Here's how the part is built. I have some questions about the finished solid (model axes, mm). A direction names the side the tool comes from. Coordinates: 2 decimals unless noted, no trailing zeros. Order: outer loops, then holes, each group sorted by start corner. A loop starts at its lowest first (then second) coordinate and runs counter-clockwise, first axis right, second up. Notation, with made-up numbers: (14.5, 13.5) - (70.5, 13.5) arc R22 ccw to (70.5, 26.5) - close; hole circle Ø10 at (26.5, -7). An arc over 180 degrees is marked (long way). Answer as CSV lines item,"result". Start each with the question number.
Q1. Suppose I cut it at B-B (x = 6). Please give me the cut outline in (y, z), then the cut area to 3 significant figures.
Q2. For faces 5 (the face through (4.5, 25, 8)), 6 (the face through (9.5, 24, 11)), 7 (the face through (13, 0, 0)), which set-ups out of +Z, -Z, +X, -X, +Y, -Y let a thin tool reach every point of the face, with its end or its side?
Q3. Suppose I cut it at A-A (x = -15). Please give me the cut outline in (y, z).
Q4. Thinking about a two-plate mould opening in Y: for faces 1 (the face through (-0.3, 8.3, -5)), 2 (the face through (0.08, 18.3, 10.51)), 3 (the face through (16.669, -30.526, -2.535)), 4 (the face through (-7, 30, 18)), which applies, released by +Y, released by -Y, zero draft, split by the parting line, or undercut?
Q5. For pin 1 Ø8.5 at (y, z) = (17.5, 20) entering from +X; pin 2 Ø11 at (y, z) = (-9.5, 18) entering from +X; pin 3 Ø5.5 at (x, z) = (-6.5, 23) entering from +Y; pin 4 Ø3 at (x, y) = (-15, 30) entering from -Z, each with a flat end and sliding along its axis, tell me the tip position at first contact or that it passes through.
Q6. I need wall thicknesses on line 1 (Y direction, x = 15, z = -2); line 2 (Z direction, x = -13, y = -27); line 3 (X direction, y = 19.5, z = 20.5). Which ranges of each line are inside material? Lowest first, please.
from build123d import *

# Parameters (mm, degrees)
SKETCH_1_W                           = 40
SKETCH_1_H                           = 70
EXTRUDE_1_DEPTH                      = 5
EXTRUDE_2_REACH                      = 92.62
EXTRUDE_START                        = -50
SKETCH_2_R                           = 12
CUT_EXTRUDE_1_REACH                  = 69.832
SKETCH_4_R                           = 1.75
FILLET_1_R                           = 3
EXTRUDE_START_2                      = 7
EXTRUDE_3_DEPTH                      = 2.5
EXTRUDE_START_3                      = -7
EXTRUDE_4_DEPTH                      = 2.5
SKETCH_5_R                           = 9.4
CUT_EXTRUDE_2_DEPTH                  = 80.580228084
CUT_EXTRUDE_3_REACH                  = 65.9
CUT_EXTRUDE_3_END_RADIUS             = 12
SKETCH_7_R                           = 1.75
CUT_EXTRUDE_3_DIRECTION_2_REACH      = 65.9
CUT_EXTRUDE_3_DIRECTION_2_END_RADIUS = 12


with BuildPart() as part:
    # ｽｹｯﾁ1 → ﾎﾞｽ - 押し出し1 (new body)
    with BuildSketch(Plane.XY):
        Rectangle(SKETCH_1_W, SKETCH_1_H)
    extrude(amount=-EXTRUDE_1_DEPTH)

    # ﾎﾞｽ - 押し出し2: up to this plane
    extrude_2_end = Plane(origin=(0, 0, 0), z_dir=(0, 0, 1))
    # ｽｹｯﾁ2 → ﾎﾞｽ - 押し出し2 (add, up to the surface)
    with BuildSketch(Plane(origin=(0, 0, 0), x_dir=(1, 0, 0), z_dir=(0, -0.49999999999999495, -0.8660254037844416)).offset(EXTRUDE_START), mode=Mode.PRIVATE) as extrude_2_sk1:
        with Locations(Location((0, 0, 0), (0, 0, 270))):
            Circle(SKETCH_2_R)
    extrude_2_tool1 = split(extrude(extrude_2_sk1.sketch, amount=EXTRUDE_2_REACH, mode=Mode.PRIVATE), bisect_by=extrude_2_end, keep=Keep.BOTH, mode=Mode.PRIVATE)
    add(extrude_2_tool1.solids().sort_by_distance((0, 25, 43.30127))[0])

    # ｽｹｯﾁ4 → ｶｯﾄ - 押し出し1 (cut, up to next)
    with BuildSketch(Plane(origin=(0, 0, -5), x_dir=(-1, 0, 0), z_dir=(0, 0, -1)), mode=Mode.PRIVATE) as cut_extrude_1_sk1:
        with Locations((-15, 30)):
            Circle(SKETCH_4_R)
    cut_extrude_1_tool1 = extrude(cut_extrude_1_sk1.sketch, amount=-CUT_EXTRUDE_1_REACH, mode=Mode.PRIVATE) & part.part
    # ｽｹｯﾁ4 → ｶｯﾄ - 押し出し1 (cut, up to next)
    with BuildSketch(Plane(origin=(0, 0, -5), x_dir=(-1, 0, 0), z_dir=(0, 0, -1)), mode=Mode.PRIVATE) as cut_extrude_1_sk2:
        with Locations(Location((15, 30, 0), (0, 0, 180))):
            Circle(SKETCH_4_R)
    cut_extrude_1_tool2 = extrude(cut_extrude_1_sk2.sketch, amount=-CUT_EXTRUDE_1_REACH, mode=Mode.PRIVATE) & part.part
    # ｽｹｯﾁ4 → ｶｯﾄ - 押し出し1 (cut, up to next)
    with BuildSketch(Plane(origin=(0, 0, -5), x_dir=(-1, 0, 0), z_dir=(0, 0, -1)), mode=Mode.PRIVATE) as cut_extrude_1_sk3:
        with Locations((15, -30)):
            Circle(SKETCH_4_R)
    cut_extrude_1_tool3 = extrude(cut_extrude_1_sk3.sketch, amount=-CUT_EXTRUDE_1_REACH, mode=Mode.PRIVATE) & part.part
    # ｽｹｯﾁ4 → ｶｯﾄ - 押し出し1 (cut, up to next)
    with BuildSketch(Plane(origin=(0, 0, -5), x_dir=(-1, 0, 0), z_dir=(0, 0, -1)), mode=Mode.PRIVATE) as cut_extrude_1_sk4:
        with Locations(Location((-15, -30, 0), (0, 0, 180))):
            Circle(SKETCH_4_R)
    cut_extrude_1_tool4 = extrude(cut_extrude_1_sk4.sketch, amount=-CUT_EXTRUDE_1_REACH, mode=Mode.PRIVATE) & part.part
    add(cut_extrude_1_tool1.solids().sort_by_distance((15, 30, -5))[0], mode=Mode.SUBTRACT)
    add(cut_extrude_1_tool2.solids().sort_by_distance((-15, 30, -5))[0], mode=Mode.SUBTRACT)
    add(cut_extrude_1_tool3.solids().sort_by_distance((-15, -30, -5))[0], mode=Mode.SUBTRACT)
    add(cut_extrude_1_tool4.solids().sort_by_distance((15, -30, -5))[0], mode=Mode.SUBTRACT)

    # ﾌｨﾚｯﾄ1
    fillet_1_edges = [part.edges().sort_by_distance(p)[0] for p in [
        (20, -35, -2.5),
        (-20, -35, -2.5),
        (-20, 35, -2.5),
        (20, 35, -2.5),
    ]]
    fillet(fillet_1_edges, radius=FILLET_1_R)

    # ｽｹｯﾁ6 → ﾎﾞｽ - 押し出し3 (add, symmetric)
    with BuildSketch(Plane(origin=(0, 0, 0), x_dir=(0, 0, -1), z_dir=(1, 0, 0)).offset(EXTRUDE_START_2)):
        Polygon((0, 30), (-38, 30), (-38, 14), (0, -30), align=None)
    extrude(amount=EXTRUDE_3_DEPTH, both=True)

    # ｽｹｯﾁ6<2> → ﾎﾞｽ - 押し出し4 (add, symmetric)
    with BuildSketch(Plane(origin=(0, 0, 0), x_dir=(0, 0, -1), z_dir=(1, 0, 0)).offset(EXTRUDE_START_3)):
        Polygon((0, 30), (-38, 30), (-38, 14), (0, -30), align=None)
    extrude(amount=EXTRUDE_4_DEPTH, both=True)

    # ｽｹｯﾁ5 → ｶｯﾄ - 押し出し2 (cut, through all)
    with BuildSketch(Plane(origin=(0, 25, 43.301270189), x_dir=(1, 0, 0), z_dir=(0, 0.49999999999999495, 0.8660254037844416))):
        with Locations(Location((0, 0, 0), (0, 0, 270))):
            Circle(SKETCH_5_R)
    extrude(amount=-CUT_EXTRUDE_2_DEPTH, mode=Mode.SUBTRACT)

    # ｶｯﾄ - 押し出し3: up to this cylinder (the profile starts inside it)
    cut_extrude_3_end = Plane(origin=(0, 14.999999951, 25.980762028), z_dir=(0, 0.4999999999999949, 0.8660254037844416)) * Cylinder(CUT_EXTRUDE_3_END_RADIUS, 176.799999934, mode=Mode.PRIVATE)
    # ｽｹｯﾁ7 → ｶｯﾄ - 押し出し3 (cut, up to the surface)
    with BuildSketch(Plane(origin=(0, 0, 0), x_dir=(1, 0, 0), z_dir=(0, 0.8660254037844416, -0.49999999999999495)), mode=Mode.PRIVATE) as cut_extrude_3_sk1:
        with Locations(Location((0, -20, 0), (0, 0, 270))):
            Circle(SKETCH_7_R)
    cut_extrude_3_tool1 = extrude(cut_extrude_3_sk1.sketch, amount=-CUT_EXTRUDE_3_REACH, mode=Mode.PRIVATE) & cut_extrude_3_end
    add(cut_extrude_3_tool1.solids().sort_by_distance((0, 10, 17.320508))[0], mode=Mode.SUBTRACT)
    # ｽｹｯﾁ7 → ｶｯﾄ - 押し出し3 (cut, up to the surface)
    with BuildSketch(Plane(origin=(0, 0, 0), x_dir=(1, 0, 0), z_dir=(0, 0.8660254037844416, -0.49999999999999495)), mode=Mode.PRIVATE) as cut_extrude_3_sk2:
        with Locations(Location((0, -40, 0), (0, 0, 270))):
            Circle(SKETCH_7_R)
    cut_extrude_3_tool2 = extrude(cut_extrude_3_sk2.sketch, amount=-CUT_EXTRUDE_3_REACH, mode=Mode.PRIVATE) & cut_extrude_3_end
    add(cut_extrude_3_tool2.solids().sort_by_distance((0, 20, 34.641016))[0], mode=Mode.SUBTRACT)

    # ｶｯﾄ - 押し出し3 direction 2: up to this cylinder (the profile starts inside it)
    cut_extrude_3_direction_2_end = Plane(origin=(0, 14.999999951, 25.980762028), z_dir=(0, 0.4999999999999949, 0.8660254037844416)) * Cylinder(CUT_EXTRUDE_3_DIRECTION_2_END_RADIUS, 176.799999934, mode=Mode.PRIVATE)
    # ｽｹｯﾁ7 → ｶｯﾄ - 押し出し3 direction 2 (cut, up to the surface)
    with BuildSketch(Plane(origin=(0, 0, 0), x_dir=(1, 0, 0), z_dir=(0, 0.8660254037844416, -0.49999999999999495)), mode=Mode.PRIVATE) as cut_extrude_3_direction_2_sk1:
        with Locations(Location((0, -20, 0), (0, 0, 270))):
            Circle(SKETCH_7_R)
    cut_extrude_3_direction_2_tool1 = extrude(cut_extrude_3_direction_2_sk1.sketch, amount=CUT_EXTRUDE_3_DIRECTION_2_REACH, mode=Mode.PRIVATE) & cut_extrude_3_direction_2_end
    add(cut_extrude_3_direction_2_tool1.solids().sort_by_distance((0, 10, 17.320508))[0], mode=Mode.SUBTRACT)
    # ｽｹｯﾁ7 → ｶｯﾄ - 押し出し3 direction 2 (cut, up to the surface)
    with BuildSketch(Plane(origin=(0, 0, 0), x_dir=(1, 0, 0), z_dir=(0, 0.8660254037844416, -0.49999999999999495)), mode=Mode.PRIVATE) as cut_extrude_3_direction_2_sk2:
        with Locations(Location((0, -40, 0), (0, 0, 270))):
            Circle(SKETCH_7_R)
    cut_extrude_3_direction_2_tool2 = extrude(cut_extrude_3_direction_2_sk2.sketch, amount=CUT_EXTRUDE_3_DIRECTION_2_REACH, mode=Mode.PRIVATE) & cut_extrude_3_direction_2_end
    add(cut_extrude_3_direction_2_tool2.solids().sort_by_distance((0, 20, 34.641016))[0], mode=Mode.SUBTRACT)


solid = part.part
Here are the results:
1,outline,"(-35, -5) - (-11.24, -5) - (18.73, 46.92) - (16, 48.5) - (5.9, 31.01) - (-30, 0) - (-35, 0) - close; (5.47, -5) - (35, -5) - (35, 0) - (30, 0) - (30, 31.18) - (34, 38.11) - (31.27, 39.68) - close"
1,area,"1,140 mm²"
2,face 5,"+Y"
2,face 6,"+X, +Y"
2,face 7,"none"
3,outline,"(-35, -5) - (-31.75, -5) - (-31.75, 0) - (-35, 0) - close; (-28.25, -5) - (28.25, -5) - (28.25, 0) - (-28.25, 0) - close; (31.75, -5) - (35, -5) - (35, 0) - (31.75, 0) - close"
4,face 1,"zero draft"
4,face 2,"undercut"
4,face 3,"undercut"
4,face 4,"released by +Y"
5,pin 1,"stops at x = 11.97"
5,pin 2,"stops at x = 9.5"
5,pin 3,"stops at y = 30"
5,pin 4,"passes through"
6,line 1,"y = -35 to -31.75, -28.25 to 28.25, 31.75 to 35"
6,line 2,"z = -5 to 0"
6,line 3,"x = -10 to -6.66, 6.66 to 10"
